from build123d import *

# Parameters (mm, degrees)
SKETCH1_W           = 57.15
SKETCH1_H           = 92.964
BOSS_EXTRUDE1_DEPTH = 1.5875
SKETCH2_R           = 1.5875
CUT_EXTRUDE1_DEPTH  = 110.137289467
SKETCH3_R           = 4.445
CUT_EXTRUDE2_DEPTH  = 110.137289467
CUT_EXTRUDE3_REACH  = 111.137


with BuildPart() as part:
    # Sketch1 → Boss-Extrude1 (new body)
    with BuildSketch(Plane(origin=(0, 0, 0), x_dir=(1, 0, 0), z_dir=(0, 1, 0))):
        with Locations((28.575, 46.482)):
            Rectangle(SKETCH1_W, SKETCH1_H)
    extrude(amount=BOSS_EXTRUDE1_DEPTH)

    # Sketch2 → Cut-Extrude1 (cut, through all)
    with BuildSketch(Plane(origin=(0, 1.5875, 0), x_dir=(1, 0, 0), z_dir=(0, 1, 0))):
        with Locations(Location((5.08, 87.884, 0), (0, 0, 270))):
            Circle(SKETCH2_R)
        with Locations(Location((52.07, 87.884, 0), (0, 0, 270))):
            Circle(SKETCH2_R)
        with Locations(Location((5.08, 5.08, 0), (0, 0, 270))):
            Circle(SKETCH2_R)
        with Locations(Location((52.07, 5.08, 0), (0, 0, 270))):
            Circle(SKETCH2_R)
    extrude(amount=-CUT_EXTRUDE1_DEPTH, mode=Mode.SUBTRACT)

    # Sketch3 → Cut-Extrude2 (cut, through all)
    with BuildSketch(Plane(origin=(0, 1.5875, 0), x_dir=(1, 0, 0), z_dir=(0, 1, 0))):
        with BuildLine():
            ThreePointArc((56.515, 46.482), (55.213089642, 43.338910358), (52.07, 42.037))
            Line((52.07, 42.037), (57.15, 42.037))
            Line((57.15, 42.037), (57.15, 50.927))
            Line((57.15, 50.927), (52.07, 50.927))
            ThreePointArc((52.07, 50.927), (55.213089642, 49.625089642), (56.515, 46.482))
        make_face()
        with Locations((52.07, 46.482)):
            Circle(SKETCH3_R)
        with Locations((5.08, 46.482)):
            Circle(SKETCH3_R)
        with BuildLine():
            Line((5.08, 50.927), (0, 50.927))
            Line((0, 50.927), (0, 42.037))
            Line((0, 42.037), (5.08, 42.037))
            ThreePointArc((5.08, 42.037), (0.635, 46.482), (5.08, 50.927))
        make_face()
    extrude(amount=-CUT_EXTRUDE2_DEPTH, mode=Mode.SUBTRACT)

    # Sketch4 → Cut-Extrude3 (cut, up to next)
    with BuildSketch(Plane(origin=(0, 1.5875, 0), x_dir=(1, 0, 0), z_dir=(0, 1, 0)), mode=Mode.PRIVATE) as cut_extrude3_sk1:
        with BuildLine():
            ThreePointArc((28.575, 3.175), (30.82006403, 4.10493597), (31.75, 6.35))
            ThreePointArc((31.75, 6.35), (30.82006403, 8.59506403), (28.575, 9.525))
            Line((28.575, 9.525), (28.575, 3.175))
        make_face()
    cut_extrude3_tool1 = extrude(cut_extrude3_sk1.sketch, amount=-CUT_EXTRUDE3_REACH, mode=Mode.PRIVATE) & part.part
    # Sketch4 → Cut-Extrude3 (cut, up to next)
    with BuildSketch(Plane(origin=(0, 1.5875, 0), x_dir=(1, 0, 0), z_dir=(0, 1, 0)), mode=Mode.PRIVATE) as cut_extrude3_sk2:
        with BuildLine():
            Line((28.575, 3.175), (28.575, 9.525))
            ThreePointArc((28.575, 9.525), (26.32993597, 8.59506403), (25.4, 6.35))
            ThreePointArc((25.4, 6.35), (26.32993597, 4.10493597), (28.575, 3.175))
        make_face()
    cut_extrude3_tool2 = extrude(cut_extrude3_sk2.sketch, amount=-CUT_EXTRUDE3_REACH, mode=Mode.PRIVATE) & part.part
    # Sketch4 → Cut-Extrude3 (cut, up to next)
    with BuildSketch(Plane(origin=(0, 1.5875, 0), x_dir=(1, 0, 0), z_dir=(0, 1, 0)), mode=Mode.PRIVATE) as cut_extrude3_sk3:
        with BuildLine():
            ThreePointArc((28.575, 3.175), (30.82006403, 4.10493597), (31.75, 6.35))
            ThreePointArc((31.75, 6.35), (30.82006403, 8.59506403), (28.575, 9.525))
            Line((28.575, 9.525), (28.575, 3.175))
        make_face()
    cut_extrude3_tool3 = extrude(cut_extrude3_sk3.sketch, amount=-CUT_EXTRUDE3_REACH, mode=Mode.PRIVATE) & part.part
    # Sketch4 → Cut-Extrude3 (cut, up to next)
    with BuildSketch(Plane(origin=(0, 1.5875, 0), x_dir=(1, 0, 0), z_dir=(0, 1, 0)), mode=Mode.PRIVATE) as cut_extrude3_sk4:
        with BuildLine():
            Line((28.575, 3.175), (28.575, 9.525))
            ThreePointArc((28.575, 9.525), (26.32993597, 8.59506403), (25.4, 6.35))
            ThreePointArc((25.4, 6.35), (26.32993597, 4.10493597), (28.575, 3.175))
        make_face()
    cut_extrude3_tool4 = extrude(cut_extrude3_sk4.sketch, amount=-CUT_EXTRUDE3_REACH, mode=Mode.PRIVATE) & part.part
    # Sketch4 → Cut-Extrude3 (cut, up to next)
    with BuildSketch(Plane(origin=(0, 1.5875, 0), x_dir=(1, 0, 0), z_dir=(0, 1, 0)), mode=Mode.PRIVATE) as cut_extrude3_sk5:
        with BuildLine():
            Line((28.575, 0), (28.575, 3.175))
            ThreePointArc((28.575, 3.175), (26.32993597, 4.10493597), (25.4, 6.35))
            Line((25.4, 6.35), (25.4, 0))
            Line((25.4, 0), (28.575, 0))
        make_face()
    cut_extrude3_tool5 = extrude(cut_extrude3_sk5.sketch, amount=-CUT_EXTRUDE3_REACH, mode=Mode.PRIVATE) & part.part
    # Sketch4 → Cut-Extrude3 (cut, up to next)
    with BuildSketch(Plane(origin=(0, 1.5875, 0), x_dir=(1, 0, 0), z_dir=(0, 1, 0)), mode=Mode.PRIVATE) as cut_extrude3_sk6:
        with BuildLine():
            Line((31.75, 0), (31.75, 6.35))
            ThreePointArc((31.75, 6.35), (30.82006403, 4.10493597), (28.575, 3.175))
            Line((28.575, 3.175), (28.575, 0))
            Line((28.575, 0), (31.75, 0))
        make_face()
    cut_extrude3_tool6 = extrude(cut_extrude3_sk6.sketch, amount=-CUT_EXTRUDE3_REACH, mode=Mode.PRIVATE) & part.part
    add(cut_extrude3_tool1.solids().sort_by_distance((29.922512, 1.5875, -6.35))[0], mode=Mode.SUBTRACT)
    add(cut_extrude3_tool2.solids().sort_by_distance((27.227488, 1.5875, -6.35))[0], mode=Mode.SUBTRACT)
    add(cut_extrude3_tool3.solids().sort_by_distance((29.922512, 1.5875, -6.35))[0], mode=Mode.SUBTRACT)
    add(cut_extrude3_tool4.solids().sort_by_distance((27.227488, 1.5875, -6.35))[0], mode=Mode.SUBTRACT)
    add(cut_extrude3_tool5.solids().sort_by_distance((26.832316, 1.5875, -1.993291))[0], mode=Mode.SUBTRACT)
    add(cut_extrude3_tool6.solids().sort_by_distance((30.317684, 1.5875, -1.993291))[0], mode=Mode.SUBTRACT)


solid = part.part
Can you work these out from the model? Positions are in its coordinate system, mm. Give positions to 0.01 mm unless a question says otherwise; leave off trailing zeros. Write each loop counter-clockwise with the first axis right and the second up, starting at its lowest first coordinate (ties: lowest second). Pieces come first, ordered by that corner, then holes. Notation, with made-up numbers: (-33, -9.75) -> (-10, -9.75) arc R22 cw to (-10, 22.25) -> close; hole circle Ø5 at (11.25, -35). An arc over 180 degrees is marked (long way). Answer as a JSON object with one key per item and string values. Group by question number.
Item 1: I'm going to push a flat-ended pin straight in: P1, Ø0.8, axis at y = 0.5, z = -2.5, coming from the -X side. Where does the tip first touch, or does it pass through?
Item 2: We'd pull the mould along Z, two halves only. Please class faces 1 (the face through (5.557, 0.805, -3.566)), 2 (the face through (28, 1.588, -47)): +Z half, -Z half, draft (parallel to the pull), parting line (faces both ways), or undercut.
Item 3: Suppose I cut it at A-A (z = -5.08). Please give me the cut outline in (x, y).
Item 4: Please list where these lines run through material, in increasing order: line 1 (X direction, y = 1.15, z = -5.08); line 2 (Z direction, x = 5, y = 1.1); line 3 (Z direction, x = 52.5, y = 0.4). Write a range as [from, to].
Item 5: Suppose I cut it at B-B (y = 0.65). State how many separate pieces and enclosed holes the cut face has, plus the area to 3 significant figures.
Findings:
{
 "1": {"P1": "stops at x = 0"},
 "2": {"face 1": "undercut", "face 2": "draft"},
 "3": {"outline": "(0, 0) -> (3.49, 0) -> (3.49, 1.59) -> (0, 1.59) -> close; (6.67, 0) -> (25.4, 0) -> (25.4, 1.59) -> (6.67, 1.59) -> close; (31.75, 0) -> (50.48, 0) -> (50.48, 1.59) -> (31.75, 1.59) -> close; (53.66, 0) -> (57.15, 0) -> (57.15, 1.59) -> (53.66, 1.59) -> close"},
 "4": {"line 1": "x = [0, 3.49], [6.67, 25.4], [31.75, 50.48], [53.66, 57.15]", "line 2": "z = [-92.96, -89.47], [-86.3, -50.93], [-42.04, -6.67], [-3.49, 0]", "line 3": "z = [-92.96, -89.41], [-86.36, -50.93], [-42.04, -6.61], [-3.55, 0]"},
 "5": {"separate pieces": "1", "enclosed holes": "4", "area": "5,070 mm²"}
}
